Geometry check sheet. Reference: the model listing, model coordinates, mm. Give positions to 0.01 mm unless a question says otherwise; leave off trailing zeros. Write each loop counter-clockwise with the first axis right and the second up, starting at its lowest first coordinate (ties: lowest second). Pieces come first, ordered by that corner, then holes. Notation, with made-up numbers: M 75,75.5 L 80,75.5 A20 cw 80,108.5 Z; hole C 68,-29.5 d6. An arc over 180 degrees is marked long. One line per item, written item: value. Start each with the question number.
1. Release check for a two-part mould opening along X. For faces 1 (the face through (22.947, 10.028, 2.218)), 2 (the face through (49.8, 25, 2)), 3 (the face through (48.15, 10.03, 2.28)), 4 (the face through (-21, 25, 4.5)) record: pulls with the +X half, pulls with the -X half, needs draft (parallel to the pull), parting line crosses it, or undercut.
2. Scan lines: line 1 (Y direction, x = 45.56, z = 1.25); line 2 (X direction, y = 4.24, z = 2.15); line 3 (Y direction, x = -39.5, z = 3.35). Record each from-to range of solid material in increasing order.
3. Cross-section at C-C on y = 22. Record the cut outline in (x, z).
4. Cross-section at A-A on x = -4.44. Record the cut outline in (y, z).
5. Cross-section at D-D on y = 38. Record the cut outline in (x, z), then the cut area to 3 significant figures.
6. Cross-section at B-B on z = 1.05. Count the separate pieces of the cut face and the enclosed holes in it, then the cut area to 3 significant figures.
Autodesk Inventor part; units mm, degrees
ref_plane "YZ Plane" through (0, 0, 0) normal (1, 0, 0) x (0, 1, 0)
ref_plane "XZ Plane" through (0, 0, 0) normal (0, 1, 0) x (-1, 0, 0)
ref_plane "XY Plane" through (0, 0, 0) normal (0, 0, 1) x (1, 0, 0)
sketch "Sketch1" plane through (0, 0, 0) normal (0, 0, 1) x (1, 0, 0)
  circle A0 centre (44.9, 4.9) radius 1.45 construction
  circle A1 centre (4.9, 4.9) radius 1.45 construction
  line L0 (2, 2) -> (2, 41.8) construction
  line L1 (47.8, 2) -> (2, 2) construction
  line L2 (47.8, 41.8) -> (47.8, 2) construction
  line L3 (41.8, 41.8) -> (47.8, 41.8) construction
  line L4 (41.8, 8) -> (41.8, 41.8) construction
  line L5 (8, 8) -> (41.8, 8) construction
  line L6 (8, 8) -> (8, 41.8) construction
  line L7 (2, 41.8) -> (8, 41.8) construction
  circle A2 centre (44.9, 44.9) radius 1.4 construction
  circle A3 centre (4.9, 44.9) radius 1.4 construction
  line L8 (2, 47.8) -> (47.8, 47.8) construction
  line L9 (2, 41.8) -> (2, 47.8) construction
  line L10 (47.8, 41.8) -> (2, 41.8) construction
  line L11 (47.8, 41.8) -> (47.8, 47.8) construction
  circle A4 centre (25.6838, 25.4066) radius 13.6 construction
  line L12 (44.1319, 49.8) -> (5.6681, 49.8) construction
  arc A5 (49.8, 47.8) -> (47.8, 49.8) centre (47.8, 47.8) ccw construction
  line L13 (49.8, 41.8) -> (49.8, 47.8) construction
  arc A6 (2, 49.8) -> (0, 47.8) centre (2, 47.8) ccw construction
  arc A7 (0, 2) -> (2, 0) centre (2, 2) ccw construction
  arc A8 (47.8, 0) -> (49.8, 2) centre (47.8, 2) ccw construction
  line L14 (49.8, 0) -> (-90.2, 0)
  line L15 (-90.2, 0) -> (-90.2, 49.8)
  line L16 (-90.2, 49.8) -> (49.8, 49.8)
  line L17 (49.8, 49.8) -> (49.8, 0)
  line L18 (8, 3.7577) -> (41.8, 3.7577) construction
  line L19 (41.8, 0) -> (41.8, 3.7577) construction
  line L20 (8, 0) -> (41.8, 0) construction
  line L21 (8, 0) -> (8, 3.7577) construction
  line L22 (46.1838, 8) -> (46.1838, 41.8) construction
  line L23 (49.8, 41.8) -> (46.1838, 41.8) construction
  line L24 (49.8, 8) -> (49.8, 41.8) construction
  line L25 (46.1838, 8) -> (49.8, 8) construction
  line L26 (3.6162, 41.8) -> (3.6162, 8) construction
  line L27 (0, 8) -> (3.6162, 8) construction
  line L28 (0, 8) -> (0, 41.8) construction
  line L29 (3.6162, 41.8) -> (0, 41.8) construction
  circle A9 centre (24.9, 24.9) radius 15
  arc A10 (42.3945, 24.4616) -> (22.4616, 42.2293) centre (24.9, 24.9) ccw construction
  arc A11 (22.5619, 16.1033) -> (42.3945, 24.4616) centre (29.0002, 28.5351) ccw construction
  line L30 (22.5619, 16.1033) -> (22.3031, 15.1374) construction
  arc A12 (22.3031, 15.1374) -> (41.5232, 19.4302) centre (29.3361, 28.8218) ccw construction
  arc A13 (15.3425, 10.2404) -> (41.5232, 19.4302) centre (24.9, 24.9) ccw construction
  arc A14 (18.2047, 31.6263) -> (15.3425, 10.2404) centre (25.6173, 19.7498) ccw construction
  line L31 (18.2047, 31.6263) -> (17.4976, 32.3335) construction
  arc A15 (17.4976, 32.3335) -> (11.1478, 14.0775) centre (25.6302, 19.2725) ccw construction
  arc A16 (16.2809, 40.1303) -> (11.1478, 14.0775) centre (24.9, 24.9) ccw construction
  arc A17 (34.0602, 27.4798) -> (16.2809, 40.1303) centre (20.0844, 26.6568) ccw construction
  line L32 (34.0602, 27.4798) -> (35.0261, 27.7386) construction
  arc A18 (35.0261, 27.7386) -> (22.4616, 42.2293) centre (19.6533, 27.1018) ccw construction
  line L33 (3.6577, 41.7) -> (8.1, 46.1423) construction
  line L34 (0, 41.7) -> (3.6577, 41.7) construction
  line L35 (0, 8.1) -> (0, 41.7) construction
  line L36 (3.6577, 8.1) -> (0, 8.1) construction
  line L37 (8.1, 3.6577) -> (3.6577, 8.1) construction
  line L38 (8.1, 0) -> (8.1, 3.6577) construction
  line L39 (41.7, 0) -> (8.1, 0) construction
  line L40 (41.7, 3.6577) -> (41.7, 0) construction
  line L41 (46.1423, 8.1) -> (41.7, 3.6577) construction
  line L42 (49.8, 8.1) -> (46.1423, 8.1) construction
  line L43 (49.8, 41.7) -> (49.8, 8.1) construction
  line L44 (46.1423, 41.7) -> (49.8, 41.7) construction
  line L45 (41.7, 46.1423) -> (46.1423, 41.7) construction
  line L46 (41.7, 49.8) -> (41.7, 46.1423) construction
  line L47 (8.1, 49.8) -> (41.7, 49.8) construction
  line L48 (8.1, 46.1423) -> (8.1, 49.8) construction
  circle A19 centre (24.9, 24.9) radius 16.9 construction
  point P0 (0, 0)
  dimension "d0" = 30
  dimension "d4" = 140
extrude "Extrusion1" add sketch "Sketch1" along normal blind 4.5
fillet "Fillet1" radius 2 4 edges at (49.8, 49.8, 2.25) (-90.2, 49.8, 2.25) (49.8, 0, 2.25) (-90.2, 0, 2.25)
sketch "Sketch2" plane through (0, 0, 0) normal (0, 0, -1) x (-1, 0, 0)
  line L0 (-41.8, 8) -> (-41.8, 41.8) construction
  line L1 (-8, 8) -> (-41.8, 8) construction
  line L2 (-8, 8) -> (-8, 41.8) construction
  line L3 (-47.8, 41.8) -> (-2, 41.8) construction
  circle A0 centre (-24.9, 24.9) radius 15 construction
  arc A1 (88.2, 0) -> (90.2, 2) centre (88.2, 2) ccw construction
  line L4 (90.2, 2) -> (90.2, 47.8) construction
  arc A2 (90.2, 47.8) -> (88.2, 49.8) centre (88.2, 47.8) ccw construction
  line L5 (88.2, 49.8) -> (-47.8, 49.8) construction
  arc A3 (-47.8, 49.8) -> (-49.8, 47.8) centre (-47.8, 47.8) ccw construction
  line L6 (-49.8, 47.8) -> (-49.8, 2) construction
  arc A4 (-49.8, 2) -> (-47.8, 0) centre (-47.8, 2) ccw construction
  line L7 (-47.8, 0) -> (88.2, 0) construction
  line L8 (-41.5, 41.5) -> (-8.3, 41.5)
  line L9 (-8.3, 41.5) -> (-8.3, 8.3)
  line L10 (-8.3, 8.3) -> (-41.5, 8.3)
  line L11 (-41.5, 8.3) -> (-41.5, 41.5)
  line L12 (-9.3, 40.5) -> (-40.5, 40.5)
  line L13 (-40.5, 40.5) -> (-40.5, 9.3)
  line L14 (-40.5, 9.3) -> (-9.3, 9.3)
  line L15 (-9.3, 9.3) -> (-9.3, 40.5)
  point P0 (0, 0)
  dimension "d6" = 0.3
  dimension "d7" = 0.3
  dimension "d8" = 0.3
  dimension "d9" = 0.3
  dimension "d10" = 1
extrude "Extrusion2" [suppressed]
sketch "Sketch4" plane through (0, 0, 0) normal (0, 0, -1) x (-1, 0, 0)
  circle A0 centre (-39.2, 45.56) radius 2.475 construction
  circle A1 centre (-10.6, 45.56) radius 2.475 construction
  circle A2 centre (-45.56, 39.2) radius 2.475 construction
  circle A3 centre (-45.56, 10.6) radius 2.475 construction
  circle A4 centre (-39.2, 4.24) radius 2.475 construction
  circle A5 centre (-4.24, 10.6) radius 2.475 construction
  circle A6 centre (-10.6, 4.24) radius 2.475 construction
  circle A7 centre (-4.24, 39.2) radius 2.475 construction
  circle A8 centre (4.44, 10.6) radius 2.475 construction
  circle A9 centre (10.8, 4.24) radius 2.475 construction
  circle A10 centre (39.4, 4.24) radius 2.475 construction
  circle A11 centre (4.44, 39.2) radius 2.475 construction
  circle A12 centre (10.8, 45.56) radius 2.475 construction
  circle A13 centre (39.4, 45.56) radius 2.475 construction
  circle A14 centre (45.76, 10.6) radius 2.475 construction
  circle A15 centre (45.76, 39.2) radius 2.475 construction
  point P0 (0, 0)
hole "Hole1" at (39.2, 45.56, 0) at (45.56, 39.2, 0) at (45.56, 10.6, 0) at (39.2, 4.24, 0) at (10.6, 45.56, 0) at (4.24, 39.2, 0) at (10.6, 4.24, 0) at (4.24, 10.6, 0) at (-4.44, 39.2, 0) at (-4.44, 10.6, 0) at (-10.8, 45.56, 0) at (-10.8, 4.24, 0) at (-39.4, 45.56, 0) at (-39.4, 4.24, 0) at (-45.76, 10.6, 0) at (-45.76, 39.2, 0) direction (0, 0, 1) diameter 5.3 end through all
equation "\"d7\" = d6"
equation "\"d8\" = d6"
equation "\"d9\" = d6"
properties part number "30_Smartphone_Holder_v3"
Report:
1. face 1: undercut
1. face 2: pulls with the +X half
1. face 3: undercut
1. face 4: needs draft
2. line 1: y = 0 to 7.95, 13.25 to 36.55, 41.85 to 49.8
2. line 2: x = -90.2 to -42.05, -36.75 to -13.45, -8.15 to 7.95, 13.25 to 36.55, 41.85 to 49.8
2. line 3: y = 0 to 1.59, 6.89 to 42.91, 48.21 to 49.8
3. outline: M -90.2,0 L 10.18,0 L 10.18,4.5 L -90.2,4.5 Z; M 39.62,0 L 49.8,0 L 49.8,4.5 L 39.62,4.5 Z
4. outline: M 0,0 L 7.95,0 L 7.95,4.5 L 0,4.5 Z; M 13.25,0 L 36.55,0 L 36.55,4.5 L 13.25,4.5 Z; M 41.85,0 L 49.8,0 L 49.8,4.5 L 41.85,4.5 Z
5. outline: M -90.2,0 L -48.12,0 L -48.12,4.5 L -90.2,4.5 Z; M -43.4,0 L -6.8,0 L -6.8,4.5 L -43.4,4.5 Z; M -2.08,0 L 1.88,0 L 1.88,4.5 L -2.08,4.5 Z; M 6.6,0 L 17.59,0 L 17.59,4.5 L 6.6,4.5 Z; M 32.21,0 L 43.2,0 L 43.2,4.5 L 32.21,4.5 Z; M 47.92,0 L 49.8,0 L 49.8,4.5 L 47.92,4.5 Z
5. area: 479 mm^2
6. separate pieces: 1
6. enclosed holes: 17
6. area: 5,910 mm^2
